Read the model definition and answer for the solid it produces. Units are mm, in the model's axes. Coordinates: 2 decimals unless noted, no trailing zeros. Order: outer loops, then holes, each group sorted by start corner. A loop starts at its lowest first (then second) coordinate and runs counter-clockwise, first axis right, second up.
Autodesk Inventor part; units mm, degrees
ref_plane "YZ Plane" through (0, 0, 0) normal (1, 0, 0) x (0, 1, 0)
ref_plane "XZ Plane" through (0, 0, 0) normal (0, 1, 0) x (-1, 0, 0)
ref_plane "XY Plane" through (0, 0, 0) normal (0, 0, 1) x (1, 0, 0)
sketch "Sketch1" plane through (0, 0, 0) normal (0, 0, 1) x (1, 0, 0)
  line L0 (-13.0592, 7.1789) -> (12.3408, 7.1789)
  line L1 (12.3408, 7.1789) -> (12.3408, -18.2211)
  line L2 (12.3408, -18.2211) -> (-13.0592, -18.2211)
  line L3 (-13.0592, -18.2211) -> (-13.0592, 7.1789)
  line L4 (10.7533, 5.5914) -> (-11.4717, 5.5914)
  line L5 (-11.4717, 5.5914) -> (-11.4717, -16.6336)
  line L6 (-11.4717, -16.6336) -> (10.7533, -16.6336)
  line L7 (10.7533, -16.6336) -> (10.7533, 5.5914)
  point P0 (0, 0)
  dimension "d0" = 25.4
  dimension "d1" = 25.4
  dimension "d2" = 1.5875
extrude "Extrusion1" add sketch "Sketch1" against normal blind 1016
properties part number "40 inch extruded alluminum tube"
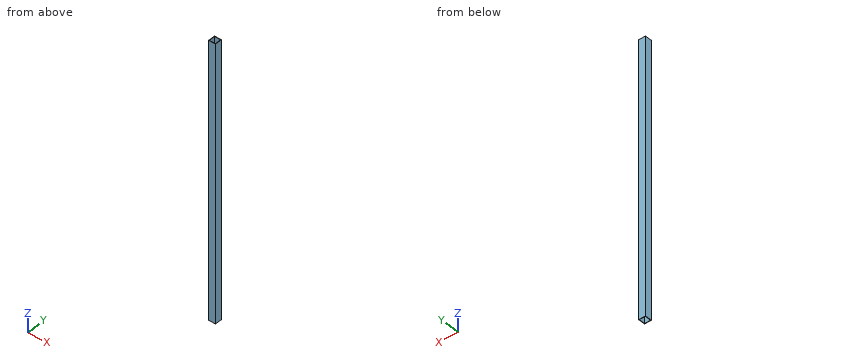
Q1. The part is cut by section A-A, the plane y = -8.5. Determine the outline of the cut face in (x, z).
Q2. The part is cut by section C-C, the plane x = -3. Determine the outline of the cut face in (y, z), then the cut area to 3 significant figures.
Q3. Straight lines are drawn through the part: L1, parallel to X at y = -13.25, z = -49; L2, parallel to Y at x = 3.5, z = -544. For each, find the intervals that lie inside material, in ascending order.
Q4. The part is cut by section B-B, the plane z = -746.5. Determine the outline of the cut face in (x, y).
Computed values:
1. outline: (-13.06, -1016) - (-11.47, -1016) - (-11.47, 0) - (-13.06, 0) - close; (10.75, -1016) - (12.34, -1016) - (12.34, 0) - (10.75, 0) - close
2. outline: (-18.22, -1016) - (-16.63, -1016) - (-16.63, 0) - (-18.22, 0) - close; (5.59, -1016) - (7.18, -1016) - (7.18, 0) - (5.59, 0) - close
2. area: 3,230 mm2
3. L1: x = -13.06 to -11.47, 10.75 to 12.34
3. L2: y = -18.22 to -16.63, 5.59 to 7.18
4. outline: (-13.06, -18.22) - (12.34, -18.22) - (12.34, 7.18) - (-13.06, 7.18) - close; hole (-11.47, -16.63) - (10.75, -16.63) - (10.75, 5.59) - (-11.47, 5.59) - close
